```python
from build123d import *

# Parameters (mm, degrees)
F1_DEPTH = 180
F2_R     = 4
F3_DEPTH = 25
F4_W     = 80
F4_H     = 50
F5_DEPTH = 12.5
F6_W     = 5.1898740767
F6_H     = 6
F7_DEPTH = 80


with BuildPart() as f1:
    # F0 (on Front) → F1 (new body)
    with BuildSketch(Plane.XZ):
        Polygon((3, 40), (0, 40), (0, 16), (-5.1898740767, 16), (-5.1898740767, 0), (-1, 0), (-1, 10), (3, 10), align=None)
        Polygon((-1, 0), (-5.1898740767, 0), (-5.1898740767, -16), (0, -16), (0, -40), (3, -40), (3, -10), (-1, -10), align=None)
    extrude(amount=F1_DEPTH)

    # F2 (on face) → F3 (cut)
    with BuildSketch(Plane(origin=(-5.1898740767, 0, 0), x_dir=(0, -1, 0), z_dir=(-1, 0, 0))):
        with Locations((170, 0)):
            Circle(F2_R)
        with Locations((155, 30)):
            Circle(F2_R)
        with Locations((105, 30)):
            Circle(F2_R)
        with Locations((155, -30)):
            Circle(F2_R)
        with Locations((105, -30)):
            Circle(F2_R)
    extrude(amount=-F3_DEPTH, mode=Mode.SUBTRACT)

    # F4 (on face) → F5 (cut, symmetric)
    with BuildSketch(Plane.YZ.offset(-1)):
        with Locations((-40, 15)):
            Rectangle(F4_W, F4_H)
    extrude(amount=F5_DEPTH, both=True, mode=Mode.SUBTRACT)

    # F6 (on face) → F7 (cut)
    with BuildSketch(Plane(origin=(0, 0, 0), x_dir=(-1, 0, 0), z_dir=(0, 1, 0))):
        with Locations((2.5949370383, -13)):
            Rectangle(F6_W, F6_H)
    extrude(amount=-F7_DEPTH, mode=Mode.SUBTRACT)


solid = f1.part
```
The model under review builds one solid part; all positions refer to its coordinate system, in mm. A direction names the side the tool comes from. Round coordinates to 2 decimals unless told otherwise and drop trailing zeros. Loops run counter-clockwise (first coordinate to the right, second up) from the corner with the lowest first, then second, coordinate; pieces in that order, holes last. Notation, with made-up numbers: (62.25, 39) - (88.25, 39) arc R12 ccw to (88.25, 45) - close; hole circle Ø3 at (1.25, -35.75). An arc over 180 degrees is marked (long way). Use a Markdown table: item, result. Add a question column.
Q1. For probe 1 along Z at (x, y) = (1.5, -171.5); probe 2 along Z at (x, y) = (-4.15, -170); probe 3 along X at (y, z) = (-170, -25.5), list the stretches that pass through material, from the lowest coordinate up.
Q2. Insertion check: pin 1 Ø7 at (y, z) = (-170, 0) entering from -X; pin 2 Ø10 at (y, z) = (-106, -4) entering from +X; pin 3 Ø9 at (y, z) = (-105, -30) entering from -X; pin 4 Ø1.6 at (x, y) = (-1.5, -115.5) entering from +Z. Each pin has a flat end and moves straight along its axis. Give the tip position at first contact, or say it passes through.
Q3. The part is to be moulded in two halves that separate along Y. For faces 5 (the face through (-1, -129, 0)), 6 (the face through (1.479, -158.815, -28.799)), 7 (the face through (-2, -80, 5)), say which applies: pulls with the +Y half, pulls with the -Y half, needs draft (parallel to the pull), parting line crosses it, or undercut.
Q4. Add section B-B (y = -170). State the section outline as (x, z) points.
Q5. Add section A-A (z = -30). State the section outline as (x, y) points.
Q6. Machinability: for faces 1 (the face through (1.479, -104.479, 33.966)), 2 (the face through (-3, -129, -16)), 3 (the face through (-3, -129, 16)), 4 (the face through (1, -91, -10)), which of the approach directions +Z, -Z, +X, -X, +Y, -Y give a long, thin tool a straight path to every point of the face, cutting with its end or side? Answer none if there is none.
Q7. Add section C-C (z = 0). State the section outline as (x, y) points.
Q8. Add section D-D (y = -105). State the section outline as (x, z) points.
Worked answers:
| question | item | result |
|---|---|---|
| 1 | probe 1 | -40 to -10, 10 to 40 |
| 1 | probe 2 | -16 to -4, 4 to 16 |
| 1 | probe 3 | 0 to 3 |
| 2 | pin 1 | through |
| 2 | pin 2 | x = -1 |
| 2 | pin 3 | x = 0 |
| 2 | pin 4 | z = 16 |
| 3 | face 5 | needs draft |
| 3 | face 6 | undercut |
| 3 | face 7 | pulls with the +Y half |
| 4 | outline | (-5.19, -16) - (0, -16) - (0, -40) - (3, -40) - (3, -10) - (-1, -10) - (-1, -4) - (-5.19, -4) - close; (-5.19, 4) - (-1, 4) - (-1, 10) - (3, 10) - (3, 40) - (0, 40) - (0, 16) - (-5.19, 16) - close |
| 5 | outline | (0, -180) - (3, -180) - (3, -159) - (0, -159) - close; (0, -151) - (3, -151) - (3, -109) - (0, -109) - close; (0, -101) - (3, -101) - (3, 0) - (0, 0) - close |
| 6 | face 1 | +X, -X |
| 6 | face 2 | -Z, -X, +Y, -Y |
| 6 | face 3 | +Z, -X, +Y, -Y |
| 6 | face 4 | +X, +Y, -Y |
| 7 | outline | (-5.19, -180) - (-1, -180) - (-1, -174) - (-5.19, -174) - close; (-5.19, -166) - (-1, -166) - (-1, -80) - (-5.19, -80) - close |
| 8 | outline | (-5.19, -16) - (0, -16) - (0, -26) - (3, -26) - (3, -10) - (-1, -10) - (-1, 10) - (3, 10) - (3, 26) - (0, 26) - (0, 16) - (-5.19, 16) - close; (0, -40) - (3, -40) - (3, -34) - (0, -34) - close; (0, 34) - (3, 34) - (3, 40) - (0, 40) - close |
